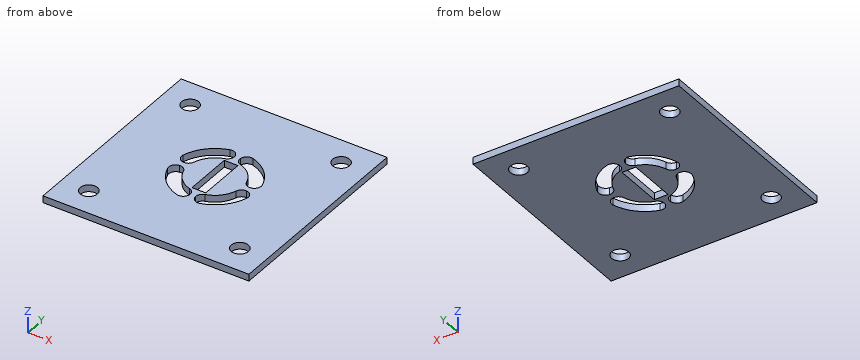
```python
from build123d import *

# Parameters (mm, degrees)
F0_W     = 38.1
F0_H     = 38.1
F1_DEPTH = 1.27
F2_R     = 1.5875
F3_DEPTH = 25.4
F6_W     = 2.54
F6_H     = 8.89
F7_DEPTH = 25.4


with BuildPart() as f1:
    # F0 (on Top) → F1 (new body)
    with BuildSketch(Plane.XY):
        Rectangle(F0_W, F0_H)
    extrude(amount=F1_DEPTH)

    # F2 (on Top) → F3 (cut)
    with BuildSketch(Plane.XY):
        with Locations((13.97, 13.97)):
            Circle(F2_R)
    extrude(amount=F3_DEPTH, mode=Mode.SUBTRACT)

    # F4: F1 across plane


with BuildPart() as f1_1:
    add(f1.part)
    add(f1.part.mirror(Plane.YZ), mode=Mode.INTERSECT)

    # F5: F1 across plane


with BuildPart() as f1_2:
    add(f1_1.part)
    add(f1_1.part.mirror(Plane.XZ), mode=Mode.INTERSECT)

    # F6 (on Top) → F7 (cut)
    with BuildSketch(Plane.XY):
        with BuildLine():
            ThreePointArc((-6.200063, -0.518475), (-7.141481, -1.065611), (-7.313076, -2.14087))
            ThreePointArc((-7.313076, -2.14087), (-5.388154, -5.388154), (-2.14087, -7.313076))
            ThreePointArc((-2.14087, -7.313076), (-1.065611, -7.141481), (-0.518475, -6.200063))
            ThreePointArc((-0.518475, -6.200063), (-0.736807, -5.375783), (-1.427246, -4.875384))
            ThreePointArc((-1.427246, -4.875384), (-3.592102, -3.592102), (-4.875384, -1.427246))
            ThreePointArc((-4.875384, -1.427246), (-5.375783, -0.736807), (-6.200063, -0.518475))
        make_face()
        with BuildLine():
            ThreePointArc((0.518475, -6.200063), (1.065611, -7.141481), (2.14087, -7.313076))
            ThreePointArc((2.14087, -7.313076), (5.388154, -5.388154), (7.313076, -2.14087))
            ThreePointArc((7.313076, -2.14087), (7.141481, -1.065611), (6.200063, -0.518475))
            ThreePointArc((6.200063, -0.518475), (5.375783, -0.736807), (4.875384, -1.427246))
            ThreePointArc((4.875384, -1.427246), (3.592102, -3.592102), (1.427246, -4.875384))
            ThreePointArc((1.427246, -4.875384), (0.736807, -5.375783), (0.518475, -6.200063))
        make_face()
        with BuildLine():
            ThreePointArc((6.200063, 0.518475), (7.141481, 1.065611), (7.313076, 2.14087))
            ThreePointArc((7.313076, 2.14087), (5.388154, 5.388154), (2.14087, 7.313076))
            ThreePointArc((2.14087, 7.313076), (1.065611, 7.141481), (0.518475, 6.200063))
            ThreePointArc((0.518475, 6.200063), (0.736807, 5.375783), (1.427246, 4.875384))
            ThreePointArc((1.427246, 4.875384), (3.592102, 3.592102), (4.875384, 1.427246))
            ThreePointArc((4.875384, 1.427246), (5.375783, 0.736807), (6.200063, 0.518475))
        make_face()
        with BuildLine():
            ThreePointArc((-0.518475, 6.200063), (-1.065611, 7.141481), (-2.14087, 7.313076))
            ThreePointArc((-2.14087, 7.313076), (-5.388154, 5.388154), (-7.313076, 2.14087))
            ThreePointArc((-7.313076, 2.14087), (-7.141481, 1.065611), (-6.200063, 0.518475))
            ThreePointArc((-6.200063, 0.518475), (-5.375783, 0.736807), (-4.875384, 1.427246))
            ThreePointArc((-4.875384, 1.427246), (-3.592102, 3.592102), (-1.427246, 4.875384))
            ThreePointArc((-1.427246, 4.875384), (-0.736807, 5.375783), (-0.518475, 6.200063))
        make_face()
        Rectangle(F6_W, F6_H)
    extrude(amount=F7_DEPTH, mode=Mode.SUBTRACT)


solid = f1_2.part
```
Part model, mm, in its own coordinate system. Round coordinates to 2 decimals unless told otherwise and drop trailing zeros. Write each loop counter-clockwise with the first axis right and the second up, starting at its lowest first coordinate (ties: lowest second). Pieces come first, ordered by that corner, then holes. Notation, with made-up numbers: M 40,-23.75 L 87,-23.75 A16 cw 87,-2.75 Z; hole C 10.5,59 d9. An arc over 180 degrees is marked long. Answer as CSV lines item,"result". Start each with the question number.
1) Band-saw the part on C-C (z = 0.35). Count the separate pieces of the cut face and the enclosed holes in it, then the cut area to 3 significant figures.
2) Drop a flat-ended pin along its axis: pin 1 (3 mm diameter, centred on x = -13.97, y = 13.97, fed in from +Z). Give the stop position or say it passes through.
3) Drill centre lines: L1, parallel to Y at x = 13.97, z = 0.85; L2, parallel to X at y = 0, z = 1.15. Where is each one in solid material? Low to high.
4) Band-saw the part on A-A (x = 13.97). List the corners of the cut face in (y, z), then the cut area to 3 significant figures.
Worked out:
1,separate pieces,"1"
1,enclosed holes,"9"
1,area,"1,310 mm²"
2,pin 1,"through"
3,L1,"-19.05 to -15.56, -12.38 to 12.38, 15.56 to 19.05"
3,L2,"-19.05 to -1.27, 1.27 to 19.05"
4,outline,"M -19.05,0 L -15.56,0 L -15.56,1.27 L -19.05,1.27 Z; M -12.38,0 L 12.38,0 L 12.38,1.27 L -12.38,1.27 Z; M 15.56,0 L 19.05,0 L 19.05,1.27 L 15.56,1.27 Z"
4,area,"40.3 mm²"
